Source: CAD feature listing. Evaluate the final solid. Frame: model axes, mm. A direction names the side the tool comes from. Round coordinates to 2 decimals unless told otherwise and drop trailing zeros. Order: outer loops, then holes, each group sorted by start corner. A loop starts at its lowest first (then second) coordinate and runs counter-clockwise, first axis right, second up. Notation, with made-up numbers: (86.25, 75) -> (131.25, 75) arc R26 ccw to (131.25, 113) -> close; hole circle Ø9 at (-7, 60). An arc over 180 degrees is marked (long way). Write item = value, one per line. Start each with the question number.
(1) Reachability of faces 1 (the face through (-6, 0, 20)), 2 (the face through (0, 2, -24)) from +Z, -Z, +X, -X, +Y, -Y: full face, straight path, thin tool, end or side. Return the list, or none.
(2) Cut plane A-A on z = 0. Return the cut outline in (x, y), then the cut area to 3 significant figures.
(3) Cut plane B-B on x = 0. Return the cut outline in (y, z).
(4) Ray query, line 1 (X direction, y = 2.9, z = 0); line 2 (Z direction, x = -16, y = 0.8); line 3 (X direction, y = 2.25, z = 18). Return the intervals inside material, ascending.
(5) Cut plane C-C on y = 2.3. Return the cut outline in (x, z), then the cut area to 3 significant figures.
(6) Draft query along Z for faces 3 (the face through (-6, 2, -22)), 4 (the face through (1.32, 2.46, -29.97)), 5 (the face through (-6, 5, 20)). Return one class per face: released by +Z, released by -Z, zero draft, split by the parting line, or undercut.
(7) Contact query for flat-ended pins moving along their axis: pin 1 Ø1 at (y, z) = (1, -16) entering from +X; pin 2 Ø1 at (y, z) = (1, 8.5) entering from +X; pin 3 Ø2 at (x, y) = (3.5, 4.5) entering from -Z; pin 4 Ø12 at (x, z) = (-7, 19) entering from -Y. Output: stop coordinate, or through.
(8) Cut plane D-D on z = 26.5. Return the cut outline in (x, y), then the cut area to 3 significant figures.
from build123d import *

# Parameters (mm, degrees)
SKIZZE1_R                       = 30
AUFSATZ_LINEAR_AUSTRAGEN1_DEPTH = 5
SKIZZE1_3_R                     = 20
SCHNITT_LINEAR_AUSTRAGEN1_DEPTH = 5
SCHNITT_LINEAR_AUSTRAGEN2_DEPTH = 5


with BuildPart() as part:
    # Skizze1 → Aufsatz-Linear austragen1 (new body)
    with BuildSketch(Plane(origin=(0, 0, 0), x_dir=(1, 0, 0), z_dir=(0, 1, 0))):
        with Locations(Location((0, 0, 0), (0, 0, 270))):  # turned: the seam where the file's is
            Circle(SKIZZE1_R)
    extrude(amount=AUFSATZ_LINEAR_AUSTRAGEN1_DEPTH)

    # Skizze1_3 → Schnitt-Linear austragen1 (cut)
    with BuildSketch(Plane(origin=(0, 0, 0), x_dir=(1, 0, 0), z_dir=(0, 1, 0))):
        with Locations(Location((0, 0, 0), (0, 0, 270))):  # turned: the seam where the file's is
            Circle(SKIZZE1_3_R)
    extrude(amount=SCHNITT_LINEAR_AUSTRAGEN1_DEPTH, mode=Mode.SUBTRACT)

    # Skizze1_4 → Schnitt-Linear austragen2 (cut)
    with BuildSketch(Plane(origin=(0, 0, 0), x_dir=(1, 0, 0), z_dir=(0, 1, 0))):
        with BuildLine():
            ThreePointArc((-6, 19.078784028), (0, 20), (6, 19.078784028))
            Line((6, 19.078784028), (6, 24))
            Line((6, 24), (-6, 24))
            Line((-6, 24), (-6, 19.078784028))
        make_face()
    extrude(amount=SCHNITT_LINEAR_AUSTRAGEN2_DEPTH, mode=Mode.SUBTRACT)


solid = part.part
Evaluation:
q1.face_1 = +Z, -Z, +X, -X, -Y
q1.face_2 = +Y, -Y
q2.outline = (-30, 0) -> (-20, 0) -> (-20, 5) -> (-30, 5) -> close; (20, 0) -> (30, 0) -> (30, 5) -> (20, 5) -> close
q2.area = 100 mm^2
q3.outline = (0, -30) -> (5, -30) -> (5, -24) -> (0, -24) -> close; (0, 20) -> (5, 20) -> (5, 30) -> (0, 30) -> close
q4.line_1 = -30 to -20, 20 to 30
q4.line_2 = -25.38 to -12, 12 to 25.38
q4.line_3 = -24 to -8.72, 8.72 to 24
q5.outline = circle Ø60 at (0, 0); hole (-6, -24) -> (6, -24) -> (6, -19.08) arc R20 ccw (long way) to (-6, -19.08) -> close
q5.area = 1,520 mm^2
q6.face_3 = undercut
q6.face_4 = split by the parting line
q6.face_5 = zero draft
q7.pin_1 = 25.69
q7.pin_2 = 28.91
q7.pin_3 = -29.9
q7.pin_4 = 0
q8.outline = (-14.06, 0) -> (14.06, 0) -> (14.06, 5) -> (-14.06, 5) -> close
q8.area = 141 mm^2
